Design review of the part built by this model. Coordinates are the model's own, in mm. Coordinates: 2 decimals unless noted, no trailing zeros. Loops run counter-clockwise (first coordinate to the right, second up) from the corner with the lowest first, then second, coordinate; pieces in that order, holes last. Notation, with made-up numbers: (42, 55.5) - (57, 55.5) arc R15 cw to (57, 63.5) - close; hole circle Ø9 at (-2.5, 86.25). An arc over 180 degrees is marked (long way). Return JSON: item names as keys, results as strings. Group by question number.
from build123d import *

# Parameters (mm, degrees)
SKETCH_1_W          = 50
SKETCH_1_H          = 80
EXTRUDE_1_DEPTH     = 3
SKETCH_2_R          = 11
SKETCH_2_R_2        = 1.25
SKETCH_2_R_3        = 1.6
CUT_EXTRUDE_1_DEPTH = 48.265209192
FILLET_1_R          = 10


with BuildPart() as part:
    # ｽｹｯﾁ1 → ﾎﾞｽ - 押し出し1 (new body)
    with BuildSketch(Plane.XY):
        Rectangle(SKETCH_1_W, SKETCH_1_H)
    extrude(amount=EXTRUDE_1_DEPTH)

    # ｽｹｯﾁ2 → ｶｯﾄ - 押し出し1 (cut, through all)
    with BuildSketch(Plane.XY.offset(3)):
        with Locations((5, 25)):
            Circle(SKETCH_2_R)
        with Locations((18.5, 24)):
            Circle(SKETCH_2_R_2)
        with Locations((-20, 35)):
            Circle(SKETCH_2_R_3)
        with Locations((-20, -25)):
            Circle(SKETCH_2_R_3)
        with Locations((-8.5, 24)):
            Circle(SKETCH_2_R_2)
        with Locations((18.5, -3)):
            Circle(SKETCH_2_R_2)
        with Locations((-20, -35)):
            Circle(SKETCH_2_R_3)
        with Locations((-10, -35)):
            Circle(SKETCH_2_R_3)
        with Locations((20, -35)):
            Circle(SKETCH_2_R_3)
        with Locations((-8.5, -3)):
            Circle(SKETCH_2_R_2)
    extrude(amount=-CUT_EXTRUDE_1_DEPTH, mode=Mode.SUBTRACT)

    # ﾌｨﾚｯﾄ1
    fillet_1_edges = [part.edges().sort_by_distance(p)[0] for p in [
        (25, 40, 1.5),
    ]]
    fillet(fillet_1_edges, radius=FILLET_1_R)


solid = part.part
Item 1: Add section C-C (z = 0.9). Give the number of separate pieces and of enclosed holes in the cut face, then the cut area to 3 significant figures.
Item 2: Add section A-A (y = -3). State the section outline as (x, z) points.
Item 3: Draft analysis for pull direction X (two halves, no side actions). For faces 1 (the face through (0, -40, 1)), 2 (the face through (-20.35, 33.44, 1.52)), 3 (the face through (25, -5, 1)), state which applies: pulls with the +X half, pulls with the -X half, needs draft (parallel to the pull), parting line crosses it, or undercut.
Item 4: To check wall thickness, follow line 1 (Y direction, x = -20, z = 1.9); line 2 (Y direction, x = 5, z = 1.75); line 3 (Y direction, x = 19, z = 1.35). State the ranges of each line that lie inside material, in increasing order. Write a range as from..to.
Item 5: For P1, Ø1.5, axis at x = -8.5, y = -3, coming from the +Z side, flat-tipped, find the tip position at first contact; note if it passes through.
Item 6: Add section D-D (x = 12.5). State the section outline as (y, z) points, then the cut area to 3 significant figures.
Item 7: Add section B-B (x = -20). State the section outline as (y, z) points.
Answers below:
{
 "1": {"separate pieces": "1", "enclosed holes": "10", "area": "3,540 mm^2"},
 "2": {"outline": "(-25, 0) - (-9.75, 0) - (-9.75, 3) - (-25, 3) - close; (-7.25, 0) - (17.25, 0) - (17.25, 3) - (-7.25, 3) - close; (19.75, 0) - (25, 0) - (25, 3) - (19.75, 3) - close"},
 "3": {"face 1": "needs draft", "face 2": "undercut", "face 3": "pulls with the +X half"},
 "4": {"line 1": "y = -40..-36.6, -33.4..-26.6, -23.4..33.4, 36.6..40", "line 2": "y = -40..14, 36..40", "line 3": "y = -40..-36.25, -33.75..-4.15, -1.85..22.85, 25.15..39.17"},
 "5": {"P1": "passes through"},
 "6": {"outline": "(-40, 0) - (16.95, 0) - (16.95, 3) - (-40, 3) - close; (33.05, 0) - (40, 0) - (40, 3) - (33.05, 3) - close", "area": "192 mm^2"},
 "7": {"outline": "(-40, 0) - (-36.6, 0) - (-36.6, 3) - (-40, 3) - close; (-33.4, 0) - (-26.6, 0) - (-26.6, 3) - (-33.4, 3) - close; (-23.4, 0) - (33.4, 0) - (33.4, 3) - (-23.4, 3) - close; (36.6, 0) - (40, 0) - (40, 3) - (36.6, 3) - close"}
}
